For this review, take the finished solid that the model builds, in its own axes (mm). A direction names the side the tool comes from. Round coordinates to 2 decimals unless told otherwise and drop trailing zeros. Order: outer loops, then holes, each group sorted by start corner. A loop starts at its lowest first (then second) coordinate and runs counter-clockwise, first axis right, second up. Notation, with made-up numbers: (22, 87) -> (28, 87) arc R24 cw to (28, 117) -> close; hole circle Ø11 at (88, 23). An arc over 180 degrees is marked (long way). Answer in a Markdown table with one row per item.
```python
from build123d import *

# Parameters (mm, degrees)
SKETCH1_R           = 13.35
SKETCH1_R_2         = 11.35
EXTRUDE_THIN1_DEPTH = 26
BOSS_EXTRUDE1_DEPTH = 5


with BuildPart() as part:
    # Sketch1 → Extrude-Thin1 (new, symmetric)
    with BuildSketch(Plane.XY):
        Circle(SKETCH1_R)
        Circle(SKETCH1_R_2, mode=Mode.SUBTRACT)
    extrude(amount=EXTRUDE_THIN1_DEPTH, both=True)

    # Sketch2 → Boss-Extrude1 (add, symmetric)
    with BuildSketch(Plane.XY):
        Polygon((15.942171509, 8.387348964), (0.707428481, 18), (-15.234743028, 9.612651036), (-15.942171509, -8.387348964), (-0.707428481, -18), (15.234743028, -9.612651036), align=None)
    extrude(amount=BOSS_EXTRUDE1_DEPTH, both=True)


solid = part.part
```
Q1. The part is to be moulded in two halves that separate along Y. For faces 1 (the face through (0, 0, 5)), 2 (the face through (7.152, -13.865, 0.07)), 3 (the face through (8, -11, -5)), say which applies: +Y half, -Y half, draft (parallel to the pull), parting line (faces both ways), or undercut.
Answer key:
| item | result |
|---|---|
| face 1 | undercut |
| face 2 | -Y half |
| face 3 | draft |
Q2. Clearance check with flat-ended pins moving along their axes: pin 1 Ø11.5 at (x, y) = (-3.5, 3) entering from -Z; pin 2 Ø7 at (x, y) = (0, 2.5) entering from +Z; pin 3 Ø4 at (x, z) = (-6.5, 13.5) entering from +Y. State where each tip first meets the part, or that it passes through.
Answer key:
| item | result |
|---|---|
| pin 1 | stops at z = -5 |
| pin 2 | stops at z = 5 |
| pin 3 | stops at y = 12.57 |
Q3. Take a section at C-C, the plane z = 4. Write out the cut boundary in (x, y), then the cut area to 3 significant figures.
Answer key:
| item | result |
|---|---|
| outline | (-15.94, -8.39) -> (-0.71, -18) -> (15.23, -9.61) -> (15.94, 8.39) -> (0.71, 18) -> (-15.23, 9.61) -> close |
| area | 843 mm^2 |
Q4. Tool access review of faces 4 (the face through (-7.152, 13.865, 0.07)), 5 (the face through (0, 0, -5)), 6 (the face through (12.734, 4.01, 15.647)): name each direction out of +Z, -Z, +X, -X, +Y, -Y from which nothing blocks a thin tool from reaching the whole face with its end or side.
Answer key:
| item | result |
|---|---|
| face 4 | +Z, -Z, -X, +Y |
| face 5 | -Z |
| face 6 | +Z |
Q5. Take a section at A-A, the plane y = 12. Write out the cut boundary in (x, z), then the cut area to 3 significant figures.
Answer key:
| item | result |
|---|---|
| outline | (-10.7, -5) -> (-5.85, -5) -> (-5.85, -26) -> (5.85, -26) -> (5.85, -5) -> (10.22, -5) -> (10.22, 5) -> (5.85, 5) -> (5.85, 26) -> (-5.85, 26) -> (-5.85, 5) -> (-10.7, 5) -> close |
| area | 701 mm^2 |
Q6. To check wall thickness, follow probe 1 along Y at (x, z) = (0, -15.25); probe 2 along X at (y, z) = (5.5, -15.5); probe 3 along X at (y, z) = (3.5, 6). State the ranges of each line that lie inside material, in increasing order.
Answer key:
| item | result |
|---|---|
| probe 1 | y = -13.35 to -11.35, 11.35 to 13.35 |
| probe 2 | x = -12.16 to -9.93, 9.93 to 12.16 |
| probe 3 | x = -12.88 to -10.8, 10.8 to 12.88 |
Q7. Take a section at B-B, the plane x = -6.5. Write out the cut boundary in (y, z), then the cut area to 3 significant figures.
Answer key:
| item | result |
|---|---|
| outline | (-14.35, -5) -> (-11.66, -5) -> (-11.66, -26) -> (-9.3, -26) -> (-9.3, -5) -> (9.3, -5) -> (9.3, -26) -> (11.66, -26) -> (11.66, -5) -> (14.21, -5) -> (14.21, 5) -> (11.66, 5) -> (11.66, 26) -> (9.3, 26) -> (9.3, 5) -> (-9.3, 5) -> (-9.3, 26) -> (-11.66, 26) -> (-11.66, 5) -> (-14.35, 5) -> close |
| area | 483 mm^2 |
Q8. Take a section at D-D, the plane z = -12. Write out the cut boundary in (x, y).
Answer key:
| item | result |
|---|---|
| outline | circle Ø26.7 at (0, 0); hole circle Ø22.7 at (0, 0) |
